from build123d import *

# Parameters (mm, degrees)
SKETCH_1_R               = 45
SKETCH_1_R_2             = 35
EXTRUDE_1_DEPTH          = 3
EXTRUDE_2_DEPTH          = 3
SKETCH_3_R               = 1.5
CUT_EXTRUDE_1_DEPTH      = 3
PATTERN_CIRCULAR_1_COUNT = 14
FILLET_1_R               = 3
EXTRUDE_3_DEPTH          = 3
FILLET_2_R               = 3
MIRROR_1_DEPTH           = 3


# Read off the part's stored shape, not the designer's step: Зеркальное отражение1
with BuildPart() as part:
    # Эскиз1 → Бобышка-Вытянуть1 (new body)
    with BuildSketch(Plane(origin=(0, 0, 0), x_dir=(1, 0, 0), z_dir=(0, 1, 0))):
        with Locations(Location((0, 0, 0), (0, 0, 270))):
            Circle(SKETCH_1_R)
        with Locations(Location((0, 0, 0), (0, 0, 270))):
            Circle(SKETCH_1_R_2, mode=Mode.SUBTRACT)
    extrude(amount=EXTRUDE_1_DEPTH)

    # Эскиз2 → Бобышка-Вытянуть2 (add)
    with BuildSketch(Plane(origin=(0, 0, 0), x_dir=(1, 0, 0), z_dir=(0, 1, 0))):
        with BuildLine():
            ThreePointArc((-34.391132578, 6.5), (-34.847450698, 3.264227303), (-35, 0))
            Line((-35, 0), (35, 0))
            ThreePointArc((35, 0), (34.847450698, 3.264227303), (34.391132578, 6.5))
            Line((34.391132578, 6.5), (-34.391132578, 6.5))
        make_face()
        with BuildLine():
            Line((35, 0), (-35, 0))
            ThreePointArc((-35, 0), (-34.847450698, -3.264227303), (-34.391132578, -6.5))
            Line((-34.391132578, -6.5), (34.391132578, -6.5))
            ThreePointArc((34.391132578, -6.5), (34.847450698, -3.264227303), (35, 0))
        make_face()
    extrude(amount=EXTRUDE_2_DEPTH)

    # Эскиз3 → Вырез-Вытянуть1 (cut)
    with BuildSketch(Plane(origin=(0, 3, 0), x_dir=(1, 0, 0), z_dir=(0, 1, 0))):
        with Locations(Location((0, 40, 0), (0, 0, 270))):
            Circle(SKETCH_3_R)
    cut_extrude_1 = extrude(amount=-CUT_EXTRUDE_1_DEPTH, mode=Mode.SUBTRACT)

    # Круговой массив1: Вырез-Вытянуть1 ×14 about axis
    pattern_circular_1_axis = Axis((0, 0, 0), (0, 1, 0))
    for i in range(1, PATTERN_CIRCULAR_1_COUNT):
        add(cut_extrude_1.rotate(pattern_circular_1_axis, i * 360 / PATTERN_CIRCULAR_1_COUNT), mode=Mode.SUBTRACT)

    # Скругление1
    fillet_1_edges = [part.edges().sort_by_distance(p)[0] for p in [
        (-34.391132578, 1.5, -6.5),
        (-34.391132578, 1.5, 6.5),
        (34.391132578, 1.5, 6.5),
        (34.391132578, 1.5, -6.5),
    ]]
    fillet(fillet_1_edges, radius=FILLET_1_R)

    # Эскиз4 → Бобышка-Вытянуть3 (add)
    with BuildSketch(Plane(origin=(0, 0, 0), x_dir=(1, 0, 0), z_dir=(0, 1, 0))):
        with BuildLine():
            Line((-3.5, 6.5), (-3.5, 34.824560299))
            ThreePointArc((-3.5, 34.824560299), (-7.551905138, 34.175557476), (-11.5, 33.056769352))
            Line((-11.5, 33.056769352), (-11.5, 6.5))
            Line((-11.5, 6.5), (-3.5, 6.5))
        make_face()
        with BuildLine():
            Line((3.5, 6.5), (3.5, 34.824560299))
            ThreePointArc((3.5, 34.824560299), (7.551905138, 34.175557476), (11.5, 33.056769352))
            Line((11.5, 33.056769352), (11.5, 6.5))
            Line((11.5, 6.5), (3.5, 6.5))
        make_face()
    extrude(amount=EXTRUDE_3_DEPTH)

    # Скругление2
    fillet_2_edges = [part.edges().sort_by_distance(p)[0] for p in [
        (-11.5, 1.5, -6.5),
        (-3.5, 1.5, -34.824560299),
        (-11.5, 1.5, -33.056769352),
        (11.5, 1.5, -6.5),
        (11.5, 1.5, -33.056769352),
        (3.5, 1.5, -34.824560299),
    ]]
    fillet(fillet_2_edges, radius=FILLET_2_R)

    # Зеркальное отражение1 outline → Зеркальное отражение1 (add)
    with BuildSketch(Plane(origin=(0, 0, 0), x_dir=(1, 0, 0), z_dir=(0, 1, 0))):
        with BuildLine():
            ThreePointArc((-0.546875, -34.995727278), (-2.637828922, -34.100775792), (-3.5, -31.996093512))
            Line((-3.5, -31.996093512), (-3.5, -6.5))
            Line((-3.5, -6.5), (-11.5, -6.5))
            Line((-11.5, -6.5), (-11.5, -28.526303651))
            ThreePointArc((-11.5, -28.526303651), (-12.93126245, -31.083462719), (-15.859375, -31.200644618))
            ThreePointArc((-15.859375, -31.200644618), (-8.419734133, -33.972166212), (-0.546875, -34.995727278))
        make_face()
        with BuildLine():
            Line((11.5, -6.5), (3.5, -6.5))
            Line((3.5, -6.5), (3.5, -31.996093512))
            ThreePointArc((3.5, -31.996093512), (2.637828922, -34.100775792), (0.546875, -34.995727278))
            ThreePointArc((0.546875, -34.995727278), (8.419734133, -33.972166212), (15.859375, -31.200644618))
            ThreePointArc((15.859375, -31.200644618), (12.93126245, -31.083462719), (11.5, -28.526303651))
            Line((11.5, -28.526303651), (11.5, -6.5))
        make_face()
    extrude(amount=MIRROR_1_DEPTH)


solid = part.part
Could you check a few things on this model? Use its own coordinates, in mm. Give positions to 0.01 mm unless a question says otherwise; leave off trailing zeros. Order: outer loops, then holes, each group sorted by start corner. A loop starts at its lowest first (then second) coordinate and runs counter-clockwise, first axis right, second up. Notation, with made-up numbers: (-38.75, -37) - (-29.75, -37) arc R8 ccw to (-29.75, -22) - close; hole circle Ø6 at (81.5, 41.5). An arc over 180 degrees is marked (long way). One line per item, written item: value. Start each with the question number.
1. For P1, Ø0.9, axis at y = 1.5, z = -23.5, coming from the +X side; P2, Ø1.5, axis at y = 0.5, z = -14, coming from the +X side; P3, Ø1.5, axis at y = 1.5, z = 18, coming from the +X side, each with a flat end and sliding along its axis, tell me the tip position at first contact or that it passes through.
2. Imagine slicing it at B-B on z = -40. List the corners of the cut face in (x, y) for me.
3. Imagine slicing it at D-D on x = 36. List the corners of the cut face in (y, z) for me, plus the area to 3 significant figures.
4. Imagine slicing it at A-A on x = -21. List the corners of the cut face in (y, z) for me, plus the area to 3 significant figures.
5. Thinking about a two-plate mould opening in Z: for faces 1 (the face through (-11.5, 1, 17)), 2 (the face through (1, 3, -1)), 3 (the face through (-17.235, 1.479, 41.569)), which applies, +Z half, -Z half, draft (parallel to the pull), parting line (faces both ways), or undercut?
6. Imagine slicing it at C-C on z = -19.5. List the corners of the cut face in (x, y) for me.
7. If I drill on probe 1 along Z at (x, y) = (-38.5, 1.6); probe 2 along X at (y, z) = (1.4, 8.5); probe 3 along X at (y, z) = (0.1, -22.5), over which ranges is the centre line in solid material (lowest first)?
Values:
1. P1: x = 38.65
1. P2: x = 43.01
1. P3: x = 41.56
2. outline: (-20.62, 0) - (-1.5, 0) - (-1.5, 3) - (-20.62, 3) - close; (1.5, 0) - (20.62, 0) - (20.62, 3) - (1.5, 3) - close
3. outline: (0, -27) - (3, -27) - (3, 27) - (0, 27) - close
3. area: 162 mm²
4. outline: (0, -39.8) - (3, -39.8) - (3, -28) - (0, -28) - close; (0, -6.5) - (3, -6.5) - (3, 6.5) - (0, 6.5) - close; (0, 28) - (3, 28) - (3, 39.8) - (0, 39.8) - close
4. area: 110 mm²
5. face 1: undercut
5. face 2: draft
5. face 3: parting line
6. outline: (-40.56, 0) - (-29.06, 0) - (-29.06, 3) - (-40.56, 3) - close; (-11.5, 0) - (-3.5, 0) - (-3.5, 3) - (-11.5, 3) - close; (3.5, 0) - (11.5, 0) - (11.5, 3) - (3.5, 3) - close; (29.06, 0) - (40.56, 0) - (40.56, 3) - (29.06, 3) - close
7. probe 1: -23.3 to -10.32, -7.49 to 7.49, 10.32 to 23.3
7. probe 2: -44.19 to -40.44, -37.55 to -33.39, -11.5 to -3.5, 3.5 to 11.5, 33.39 to 37.55, 40.44 to 44.19
7. probe 3: -38.97 to -26.81, -11.5 to -3.5, 3.5 to 11.5, 26.81 to 38.97
